```python
from build123d import *

# Parameters (mm, degrees)
SKETCH039_W      = 60
SKETCH039_H      = 74
SKETCH039_R      = 1.25
SKETCH039_W_2    = 8
SKETCH039_H_2    = 8
EXTRUDE040_DEPTH = 1


with BuildPart() as bevel001:
    # Sweep002: sweep along a path in Sketch041
    with BuildLine(Plane(origin=(0, 0, -2), x_dir=(1, 0, 0), z_dir=(0, 0, -1))) as sweep002_path:
        Line((-25, 35), (25, 35))
        ThreePointArc((25, 35), (27.12132, 34.12132), (28, 32))
        Line((28, 32), (28, -32))
        ThreePointArc((28, -32), (27.12132, -34.12132), (25, -35))
        Line((25, -35), (-25, -35))
        ThreePointArc((-25, -35), (-27.12132, -34.12132), (-28, -32))
        Line((-28, -32), (-28, 32))
        ThreePointArc((-28, 32), (-27.12132, 34.12132), (-25, 35))
    # Sketch040 → Sweep002 (sweep)
    with BuildSketch(Plane.XZ):
        Polygon((-28, 11), (-30, 9), (-30, 1), (-28, -1), (-28, -2), (-33, -2), (-33, 12), (-28, 12), align=None)
    sweep(path=sweep002_path.line)


with BuildPart() as cut026:
    # Sketch039 → Extrude040 (new body)
    with BuildSketch(Plane.XY):
        Rectangle(SKETCH039_W, SKETCH039_H)
        with Locations((-25, 32)):
            Circle(SKETCH039_R, mode=Mode.SUBTRACT)
        with Locations((25, 32)):
            Circle(SKETCH039_R, mode=Mode.SUBTRACT)
        with Locations((-25, -32)):
            Circle(SKETCH039_R, mode=Mode.SUBTRACT)
        with Locations((25, -32)):
            Circle(SKETCH039_R, mode=Mode.SUBTRACT)
        with Locations((17, 30)):
            Rectangle(SKETCH039_W_2, SKETCH039_H_2, mode=Mode.SUBTRACT)
    extrude(amount=-EXTRUDE040_DEPTH)

    # Cut026: cut bevel001
    add(bevel001.part, mode=Mode.SUBTRACT)


solid = cut026.part
```
Geometry: final body of the model. Coordinates: model frame, mm. Coordinates: 2 decimals unless noted, no trailing zeros. Order: outer loops, then holes, each group sorted by start corner. A loop starts at its lowest first (then second) coordinate and runs counter-clockwise, first axis right, second up. Notation, with made-up numbers: (49.5, -0.5) - (57.5, -0.5) arc R31 cw to (57.5, 34.5) - close; hole circle Ø10 at (1, -31). An arc over 180 degrees is marked (long way). Write each question's results on one line, items separated by ' | '.
(1) Section query A-A, the plane y = 27. Return the cut outline in (x, z).
Values found:
outline: (-29, 0) - (-28, -1) - (13, -1) - (13, 0) - close; (21, -1) - (28, -1) - (29, 0) - (21, 0) - close
(2) Section query C-C, the plane y = -16.5. Return the cut outline in (x, z), plus the area to 3 significant figures.
Values found:
outline: (-29, 0) - (-28, -1) - (28, -1) - (29, 0) - close | area: 57.0 mm²
(3) First-contact query: pin 1 Ø1.5 at (x, y) = (-25, 32) entering from +Z. Flat tip, straight axial feed; report the tip coordinate or a pass-through.
Values found:
pin 1: passes through
(4) Section query B-B, the plane z = -0.6. Return the cut outline in (x, y).
Values found:
outline: (-28.4, -32) arc R3.4 ccw to (-25, -35.4) - (25, -35.4) arc R3.4 ccw to (28.4, -32) - (28.4, 32) arc R3.4 ccw to (25, 35.4) - (-25, 35.4) arc R3.4 ccw to (-28.4, 32) - close; hole circle Ø2.5 at (-25, -32); hole circle Ø2.5 at (-25, 32); hole (13, 26) - (21, 26) - (21, 34) - (13, 34) - close; hole circle Ø2.5 at (25, -32); hole circle Ø2.5 at (25, 32)
(5) Line query: line 1 (Y direction, x = 25, z = -0.7). Output: solid intervals per line, ascending. Write a range as [from, to].
Values found:
line 1: y = [-35.3, -33.25], [-30.75, 30.75], [33.25, 35.3]
(6) Mould query, pull axis Y, two halves, no side actions, for faces 1 (the face through (0, 1, 0)), 2 (the face through (27.348, 34.297, -0.715)), 3 (the face through (26.155, 31.521, -0.493)). Classes: +Y half, -Y half, draft (parallel to the pull), parting line (faces both ways), or undercut.
Values found:
face 1: draft | face 2: +Y half | face 3: undercut
